Could you check a few things on this model? Use its own coordinates, in mm. A direction names the side the tool comes from. Coordinates: 2 decimals unless noted, no trailing zeros. Order: outer loops, then holes, each group sorted by start corner. A loop starts at its lowest first (then second) coordinate and runs counter-clockwise, first axis right, second up.
```python
from build123d import *

# Parameters (mm, degrees)
PAD_DEPTH       = 8
FILLET_R        = 1.5
POCKET_DEPTH    = 7
POCKET001_DEPTH = 10
POCKET002_DEPTH = 10


with BuildPart() as part:
    # Sketch → Pad (new body)
    with BuildSketch(Plane.XY):
        with BuildLine():
            Line((-19.5, 18.25), (-19.5, -18.25))
            ThreePointArc((-19.5, -18.25), (-18.767767, -20.017767), (-17, -20.75))
            Line((-17, -20.75), (17, -20.75))
            ThreePointArc((17, -20.75), (18.767767, -20.017767), (19.5, -18.25))
            Line((19.5, -18.25), (19.5, 18.25))
            ThreePointArc((19.5, 18.25), (18.767767, 20.017767), (17, 20.75))
            Line((17, 20.75), (-17, 20.75))
            ThreePointArc((-17, 20.75), (-18.767767, 20.017767), (-19.5, 18.25))
        make_face()
    extrude(amount=PAD_DEPTH)

    # Fillet
    fillet_edges = [part.edges().sort_by_distance(p)[0] for p in [
        (-19.5, 0, 8),
        (-18.767767, -20.017767, 8),
        (0, -20.75, 8),
        (18.767767, -20.017767, 8),
        (19.5, 0, 8),
        (18.767767, 20.017767, 8),
        (0, 20.75, 8),
        (-18.767767, 20.017767, 8),
    ]]
    fillet(fillet_edges, radius=FILLET_R)

    # Sketch001 (on Face4 of Fillet) → Pocket (cut)
    with BuildSketch(Plane(origin=(0, 0, 0), x_dir=(1, 0, 0), z_dir=(0, 0, -1))):
        with BuildLine():
            Line((-18.75, 17), (-18.75, -17))
            ThreePointArc((-18.75, -17), (-17.87132, -19.12132), (-15.75, -20))
            Line((-15.75, -20), (15.75, -20))
            ThreePointArc((15.75, -20), (17.87132, -19.12132), (18.75, -17))
            Line((18.75, -17), (18.75, 17))
            ThreePointArc((18.75, 17), (17.87132, 19.12132), (15.75, 20))
            Line((15.75, 20), (-15.75, 20))
            ThreePointArc((-15.75, 20), (-17.87132, 19.12132), (-18.75, 17))
        make_face()
    extrude(amount=-POCKET_DEPTH, mode=Mode.SUBTRACT)

    # Sketch003 → Pocket001 (cut)
    with BuildSketch(Plane.XY):
        with BuildLine():
            Line((-15, 20.25), (-15, 17.25))
            ThreePointArc((-15, 17.25), (-14.707107, 16.542893), (-14, 16.25))
            Line((-14, 16.25), (14, 16.25))
            ThreePointArc((14, 16.25), (14.707107, 16.542893), (15, 17.25))
            Line((15, 17.25), (15, 20.25))
            ThreePointArc((15, 20.25), (14.707107, 20.957107), (14, 21.25))
            Line((14, 21.25), (-14, 21.25))
            ThreePointArc((-14, 21.25), (-14.707107, 20.957107), (-15, 20.25))
        make_face()
    extrude(amount=POCKET001_DEPTH, mode=Mode.SUBTRACT)

    # Sketch004 → Pocket002 (cut)
    with BuildSketch(Plane.XY):
        with BuildLine():
            Line((-15, -16.75), (-15, -19.75))
            ThreePointArc((-15, -19.75), (-14.707107, -20.457107), (-14, -20.75))
            Line((-14, -20.75), (13.998937, -20.75))
            ThreePointArc((13.998937, -20.75), (14.706044, -20.457107), (14.998937, -19.75))
            Line((14.998937, -19.75), (14.998937, -17.002513))
            ThreePointArc((14.998937, -17.002513), (14.632085, -16.116853), (13.746424, -15.75))
            Line((13.746424, -15.75), (-14, -15.75))
            ThreePointArc((-14, -15.75), (-14.707107, -16.042893), (-15, -16.75))
        make_face()
    extrude(amount=POCKET002_DEPTH, mode=Mode.SUBTRACT)


solid = part.part
```
Item 1: Suppose I cut it at B-B (y = -3.5). List the corners of the cut face in (x, z) for me.
Item 2: For pin 1 Ø0.8 at (y, z) = (-18, 7.5) entering from -X; pin 2 Ø8 at (x, y) = (7.5, -16.5) entering from -Z; pin 3 Ø1.5 at (x, z) = (3.5, 6) entering from -Y; pin 4 Ø0.5 at (x, z) = (1.5, 7.5) entering from -Y, each with a flat end and sliding along its axis, tell me the tip position at first contact or that it passes through.
Item 3: Suppose I cut it at C-C (x = -13.5). List the corners of the cut face in (y, z) for me.
Item 4: Thinking about a two-plate mould opening in X: for faces 1 (the face through (0.1, -15.75, 7.5)), 2 (the face through (-19, 0, 0)), 3 (the face through (18.748, -20.037, 3.204)), which applies, +X half, -X half, draft (parallel to the pull), parting line (faces both ways), or undercut?
Item 5: Which directions (+Z, -Z, +X, -X, +Y, -Y) give clear straight access to the entire face, cutting with the end or side of a thin tool? Please do faces 4 (the face through (-17.89, 19.1, 3.45)), 5 (the face through (-16, 20.75, 3)), 6 (the face through (-0.2, 16.25, 7.5)), 7 (the face through (15.85, -20.32, 7.55)), 8 (the face through (14.642, -16.127, 7.493)).
Item 6: Suppose I cut it at A-A (z = 5). List the corners of the cut face in (x, y) for me, and give its area (3 significant figures).
Item 7: I need wall thicknesses on line 1 (X direction, y = -10, z = 1.5); line 2 (Y direction, x = 16, z = 3.5); line 3 (Z direction, x = -14.5, y = -11.5). Which ranges of each line are inside material? Lowest first, please.
Geometry results:
1. outline: (-19.5, 0) - (-18.75, 0) - (-18.75, 7) - (18.75, 7) - (18.75, 0) - (19.5, 0) - (19.5, 6.5) arc R1.5 ccw to (18, 8) - (-18, 8) arc R1.5 ccw to (-19.5, 6.5) - close
2. pin 1: stops at x = -19.37
2. pin 2: stops at z = 7
2. pin 3: passes through
2. pin 4: stops at y = -15.75
3. outline: (-15.75, 7) - (16.25, 7) - (16.25, 8) - (-15.75, 8) - close
4. face 1: undercut
4. face 2: draft
4. face 3: +X half
5. face 4: -Z
5. face 5: +Z, -Z, +X, -X, +Y
5. face 6: +Z, -Z, +Y
5. face 7: +Z, +X, -X, -Y
5. face 8: +Z, -Z
6. outline: (-19.5, -18.25) arc R2.5 ccw to (-17, -20.75) - (-14, -20.75) arc R1 cw to (-14.97, -20) - (-15.75, -20) arc R3 cw to (-18.75, -17) - (-18.75, 17) arc R3 cw to (-15.75, 20) - (-15, 20) - (-15, 20.25) arc R1 cw to (-14.87, 20.75) - (-17, 20.75) arc R2.5 ccw to (-19.5, 18.25) - close; (14, -20.75) - (17, -20.75) arc R2.5 ccw to (19.5, -18.25) - (19.5, 18.25) arc R2.5 ccw to (17, 20.75) - (14.87, 20.75) arc R1 cw to (15, 20.25) - (15, 20) - (15.75, 20) arc R3 cw to (18.75, 17) - (18.75, -17) arc R3 cw to (15.75, -20) - (14.97, -20) arc R1 cw to start
6. area: 76.3 mm2
7. line 1: x = -19.5 to -18.75, 18.75 to 19.5
7. line 2: y = -20.75 to -19.99, 19.99 to 20.75
7. line 3: z = 7 to 8
